Build history of the part. All positions in model axes, mm. A direction names the side the tool comes from. Round coordinates to 2 decimals unless told otherwise and drop trailing zeros. Write each loop counter-clockwise with the first axis right and the second up, starting at its lowest first coordinate (ties: lowest second). Pieces come first, ordered by that corner, then holes. Notation, with made-up numbers: (31.5, -32.5) - (45.5, -32.5) arc R25 cw to (45.5, -17.5) - close; hole circle Ø1 at (-13, -18). An arc over 180 degrees is marked (long way). One line per question, with ' | ' between items.
Autodesk Inventor part; units mm, degrees
ref_plane "YZ Plane" through (0, 0, 0) normal (1, 0, 0) x (0, 1, 0)
ref_plane "XZ Plane" through (0, 0, 0) normal (0, 1, 0) x (-1, 0, 0)
ref_plane "XY Plane" through (0, 0, 0) normal (0, 0, 1) x (1, 0, 0)
sketch "Sketch1" plane through (0, 0, 0) normal (0, 0, 1) x (1, 0, 0)
  line L0 (-50, 75) -> (50, 75)
  line L1 (50, 75) -> (50, -75)
  line L2 (50, -75) -> (-50, -75)
  line L3 (-50, -75) -> (-50, 75)
  line L4 (-50, 75) -> (-45, 75)
  line L5 (-45, 75) -> (-45, 50)
  line L6 (-45, 50) -> (-50, 50)
  line L7 (-50, 50) -> (-50, 75)
  line L8 (-50, 50) -> (-45, 50)
  line L9 (-45, 50) -> (-45, 30)
  line L10 (-45, 30) -> (-50, 30)
  line L11 (-50, 30) -> (-50, 50)
  line L12 (-45, 30) -> (-50, 30)
  line L13 (-50, 30) -> (-50, 11)
  line L14 (-50, 11) -> (-45, 11)
  line L15 (-45, 11) -> (-45, 30)
  line L16 (-50, 11) -> (-45, 11)
  line L17 (-45, 11) -> (-45, -9)
  line L18 (-45, -9) -> (-50, -9)
  line L19 (-50, -9) -> (-50, 11)
  line L20 (-50, -9) -> (-45, -9)
  line L21 (-45, -9) -> (-45, -28)
  line L22 (-45, -28) -> (-50, -28)
  line L23 (-50, -28) -> (-50, -9)
  line L24 (-45, -28) -> (-50, -28)
  line L25 (-50, -28) -> (-50, -48)
  line L26 (-50, -48) -> (-45, -48)
  line L27 (-45, -48) -> (-45, -28)
  line L28 (-50, -48) -> (-45, -48)
  line L29 (-45, -48) -> (-45, -67)
  line L30 (-50, -67) -> (-50, -48)
  line L31 (-45, -67) -> (-45, -75)
  line L32 (-45, -75) -> (-50, -75)
  line L33 (-50, -75) -> (-50, -67)
  line L34 (-45, 75) -> (-25, 75)
  line L35 (-25, 75) -> (-25, 70)
  line L36 (-25, 70) -> (-45, 70)
  line L37 (-45, 70) -> (-45, 75)
  line L38 (-25, 70) -> (-6, 70)
  line L39 (-6, 70) -> (-6, 75)
  line L40 (-6, 75) -> (-25, 75)
  line L41 (-25, 75) -> (-25, 70)
  line L42 (-6, 70) -> (14, 70)
  line L43 (14, 70) -> (14, 75)
  line L44 (14, 75) -> (-6, 75)
  line L45 (-6, 75) -> (-6, 70)
  line L46 (14, 70) -> (33, 70)
  line L47 (33, 70) -> (33, 75)
  line L48 (33, 75) -> (14, 75)
  line L49 (14, 75) -> (14, 70)
  line L50 (33, 70) -> (50, 70)
  line L51 (50, 70) -> (50, 75)
  line L52 (50, 75) -> (33, 75)
  line L53 (33, 75) -> (33, 70)
  line L54 (50, 75) -> (53, 75)
  line L55 (53, 75) -> (53, 70)
  line L56 (53, 70) -> (50, 70)
  line L57 (50, 70) -> (50, 75)
  line L58 (53, 70) -> (53, -75)
  line L59 (53, -75) -> (50, -75)
  line L60 (0, 0) -> (92.6837, 0)
  line L61 (92.6837, 0) -> (-105.3184, 0)
  line L62 (53, -75) -> (33, -75)
  line L63 (33, -75) -> (33, -70)
  line L64 (33, -70) -> (53, -70)
  line L65 (53, -70) -> (53, -75)
  line L66 (33, -70) -> (14, -70)
  line L67 (14, -70) -> (14, -75)
  line L68 (14, -75) -> (33, -75)
  line L69 (33, -75) -> (33, -70)
  line L70 (14, -75) -> (-6, -75)
  line L71 (-6, -75) -> (-6, -70)
  line L72 (-6, -70) -> (14, -70)
  line L73 (14, -70) -> (14, -75)
  line L74 (-6, -75) -> (-25, -75)
  line L75 (-25, -75) -> (-25, -70)
  line L76 (-25, -70) -> (-6, -70)
  line L77 (-6, -70) -> (-6, -75)
  line L78 (-25, -75) -> (-45, -75)
  line L79 (-45, -75) -> (-45, -70)
  line L80 (-45, -70) -> (-25, -70)
  line L81 (-25, -70) -> (-25, -75)
  dimension "d0" = 100
  dimension "d1" = 150
  dimension "d2" = 75
  dimension "d3" = 50
  dimension "d4" = 5
  dimension "d5" = 25
  dimension "d6" = 20
  dimension "d7" = 19
  dimension "d8" = 20
  dimension "d9" = 19
  dimension "d10" = 20
  dimension "d11" = 19
  dimension "d12" = 20
  dimension "d13" = 5
  dimension "d14" = 19
  dimension "d15" = 20
  dimension "d16" = 19
  dimension "d17" = 17
  dimension "d18" = 3
  dimension "d19" = 20
  dimension "d20" = 5
  dimension "d21" = 19
  dimension "d22" = 20
  dimension "d23" = 19
extrude "Extrusion1" add sketch "Sketch1" along normal blind 5 contours L0 L35 L36 L5 | L6 L9 L10 L3 | L36 L38 L42 L46 L50 L1 L60 L61 L17 L15 L9 L5 | L0 L43 L42 L39 | L14 L17 L61 L3 | L61 L17 L18 L3 | L0 L1 L50 L47 | L61 L60 L1 L64 L66 L72 L76 L80 L31 L29 L27 L21 L17 | L54 L55 L56 L1 | L22 L27 L26 L3 | L56 L58 L60 L1 | L60 L58 L64 L1 | L64 L58 L59 L1 | L1 L2 L63 L64 | L31 L80 L75 L2 | L67 L2 L71 L72
Q1. Drill centre lines: L1, parallel to X at y = -68, z = 4.7; L2, parallel to Y at x = -15, z = 4.5. Where is each one in solid material? Low to high. Write a range as from..to.
Found:
L1: -45..53 | L2: -70..70
Q2. Drop flat-ended pins along their axis: pin 1 (2.5 mm diameter, centred on y = -22.5, z = 2.5, fed in from -X); pin 2 (2.5 mm diameter, centred on x = -48, z = 2, fed in from +Y); pin 3 (1 mm diameter, centred on x = -12.5, z = 1.5, fed in from -Y). Give the stop position or say it passes through.
Found:
pin 1: x = -45 | pin 2: y = 50 | pin 3: y = -70
Q3. Saw through at B-B, the plane y = 15. List the corners of the cut face in (x, z), then the cut area to 3 significant figures.
Found:
outline: (-45, 0) - (53, 0) - (53, 5) - (-45, 5) - close | area: 490 mm^2
Q4. Saw through at C-C, the plane x = -9. List the corners of the cut face in (y, z), then the cut area to 3 significant figures.
Found:
outline: (-70, 0) - (70, 0) - (70, 5) - (-70, 5) - close | area: 700 mm^2
Q5. Which spindle directions (+Z, -Z, +X, -X, +Y, -Y) get a long thin tool onto all of the face, cutting with end or side? Do faces 1 (the flat face through (14, 72, 2)), 2 (the flat face through (-47, 50, 2)), 3 (the flat face through (-48, 11, 2)), 4 (the flat face through (-45, -61, 2)), 5 (the flat face through (14, -72, 2)). Say none if no direction does.
Found:
face 1: +Z, -Z, +Y | face 2: +Z, -Z, -X, +Y | face 3: +Z, -Z, -X | face 4: +Z, -Z, -X, -Y | face 5: +Z, -Z, -Y
